Could you check a few things on this model? Use its own coordinates, in mm. A direction names the side the tool comes from. Round coordinates to 2 decimals unless told otherwise and drop trailing zeros. Write each loop counter-clockwise with the first axis right and the second up, starting at its lowest first coordinate (ties: lowest second). Pieces come first, ordered by that corner, then holes. Notation, with made-up numbers: (37.5, -28) - (92.5, -28) arc R30 cw to (92.5, -1) - close; hole circle Ø6 at (34.5, 34). An arc over 180 degrees is marked (long way). Write each question's results on one line, items separated by ' | '. Start each with the question number.
(1) Imagine slicing it at A-A on y = 7. Write out the boundary of the cut face in (x, z).
(2) Imagine slicing it at D-D on y = 15. Write out the boundary of the cut face in (x, z).
(3) Please list where these lines run through material, in increasing order: line 1 (Y direction, x = 11.2, z = 0); line 2 (X direction, y = 21.8, z = 0); line 3 (Z direction, x = 0, y = 22.15). Write a range as [from, to].
(4) On a 3-axis mill with a long thin cutter (end or side, diameter ignored), from which of +Z, -Z, +X, -X, +Y, -Y can I reach the whole of each face in a straight line? I mean faces 1 (the cylindrical face through (10.479, 18.584, -0.314)), 2 (the flat face through (-7, 18, 3)), 3 (the cylindrical face through (11.699, 11.325, 7.815)), 4 (the flat face through (3, 2, -3)), 5 (the flat face through (8, 21, -2.65)). Say none if no direction works.
(5) Thinking about a two-plate mould opening in X: for faces 6 (the flat face through (6, 10, -4)), 7 (the flat face through (5.568, 2.986, -3.155)), 8 (the flat face through (2, 16, 0)), which applies, +X half, -X half, draft (parallel to the pull), parting line (faces both ways), or undercut?
(6) Imagine slicing it at B-B on x = 8. Write out the boundary of the cut face in (y, z).
(7) For P1, Ø0.6, axis at y = 2.5, z = -1.5, coming from the +X side; P2, Ø2.5, axis at y = 19, z = 0.5, coming from the -X side; P3, Ø0.6, axis at x = -6, y = 18.5, coming from the -Z side, each with a flat end and sliding along its axis, tell me the tip position at first contact or that it passes through.
(8) Imagine slicing it at C-C on z = 3. State how many separate pieces and enclosed holes the cut face has, then the cut area to 3 significant figures.
```python
from build123d import *

# Parameters (mm, degrees)
SKETCH1_W                  = 12
SKETCH1_H                  = 13
BOSS_EXTRUDE1_DEPTH        = 19
SKETCH2_R                  = 4
CUT_EXTRUDE1_DEPTH         = 16
CUT_EXTRUDE2_START         = -2
SKETCH3_W                  = 12
SKETCH3_H                  = 13
CUT_EXTRUDE2_DEPTH         = 6
SKETCH5_W                  = 12
SKETCH5_H                  = 13
BOSS_EXTRUDE2_DEPTH        = 5
FILLET1_R                  = 2
FILLET4_R                  = 2
SKETCH21_W                 = 2.5
SKETCH21_H                 = 8
SKETCH21_W_2               = 9
SKETCH21_H_2               = 1.5
BOSS_EXTRUDE4_DEPTH        = 1
FILLET3_R                  = 0.5
FILLET7_R                  = 0.5
FILLET5_R                  = 0.5
SKETCH23_R                 = 4
BOSS_EXTRUDE5_DEPTH        = 1
BOSS_EXTRUDE6_DEPTH        = 13
BOSS_EXTRUDE7_DEPTH        = 25
SKETCH11_W                 = 2.3
SKETCH11_H                 = 5.3
CUT_EXTRUDE4_DEPTH         = 7
SKETCH34_W                 = 13.5
SKETCH34_H                 = 6
CUT_EXTRUDE5_DEPTH         = 15
M2_5_CLEARANCE_HOLE1_D     = 2.9
M2_5_CLEARANCE_HOLE1_DEPTH = 13.378752102
M2_5_CLEARANCE_HOLE1_TIP   = 0.871247898
FILLET8_R                  = 0.4
SKETCH31_R                 = 3.625
SKETCH31_R_2               = 2.625
BOSS_EXTRUDE8_DEPTH        = 2.75
FILLET9_R                  = 1
SKETCH9_R                  = 1
CUT_EXTRUDE6_DEPTH         = 29.889617512
CUT_EXTRUDE8_DEPTH         = 12
FILLET10_R                 = 5
BOSS_EXTRUDE9_DEPTH        = 2


with BuildPart() as part:
    # Sketch1 → Boss-Extrude1 (new body)
    with BuildSketch(Plane(origin=(0, 0, 0), x_dir=(1, 0, 0), z_dir=(0, 1, 0))):
        Rectangle(SKETCH1_W, SKETCH1_H)
    extrude(amount=BOSS_EXTRUDE1_DEPTH)

    # Sketch2 → Cut-Extrude1 (cut)
    with BuildSketch(Plane.XZ):
        with Locations(Location((0, 0, 0), (0, 0, 270))):
            Circle(SKETCH2_R)
    extrude(amount=-CUT_EXTRUDE1_DEPTH, mode=Mode.SUBTRACT)

    # Sketch3 → Cut-Extrude2 (cut)
    with BuildSketch(Plane.XZ.offset(CUT_EXTRUDE2_START)):
        Rectangle(SKETCH3_W, SKETCH3_H)
    extrude(amount=-CUT_EXTRUDE2_DEPTH, mode=Mode.SUBTRACT)


with BuildPart() as cut_extrude2_piece_1:
    # of the separate pieces the step leaves, piece 1, a body of its own (cut_extrude2_pieces)
    add(part.part.solids().sort_by_distance((-6, 8, 6.5))[0])

    # Sketch5 → Boss-Extrude2 (add)
    with BuildSketch(Plane(origin=(0, 19, 0), x_dir=(1, 0, 0), z_dir=(0, 1, 0))):
        Rectangle(SKETCH5_W, SKETCH5_H)
    extrude(amount=BOSS_EXTRUDE2_DEPTH)

    # Fillet1
    fillet1_edges = [cut_extrude2_piece_1.edges().sort_by_distance(p)[0] for p in [
        (-6, 16, -6.5),
        (-6, 16, 6.5),
    ]]
    fillet(fillet1_edges, radius=FILLET1_R)



with BuildPart() as cut_extrude2_piece_2:
    # of the separate pieces the step leaves, piece 2, a body of its own (cut_extrude2_pieces)
    add(part.part.solids().sort_by_distance((-6, 0, 6.5))[0])

    # Fillet4
    fillet4_edges = [cut_extrude2_piece_2.edges().sort_by_distance(p)[0] for p in [
        (-6, 1, 6.5),
        (-6, 1, -6.5),
    ]]
    fillet(fillet4_edges, radius=FILLET4_R)

    # Sketch21 → Boss-Extrude4 (add)
    with BuildSketch(Plane.ZY.offset(6)):
        with Locations((-3.25, 18)):
            Rectangle(SKETCH21_W, SKETCH21_H)
        with Locations((3.25, 18)):
            Rectangle(SKETCH21_W, SKETCH21_H)
        with Locations((0, 0.75)):
            Rectangle(SKETCH21_W_2, SKETCH21_H_2)
    extrude(amount=BOSS_EXTRUDE4_DEPTH)


with BuildPart() as boss_extrude4_piece_1:
    # of the separate pieces the step leaves, piece 1, a body of its own (boss_extrude4_pieces)
    add(cut_extrude2_piece_2.part.solids().sort_by_distance((-4, 0, 6.5))[0])

    # Fillet5
    fillet5_edges = [boss_extrude4_piece_1.edges().sort_by_distance(p)[0] for p in [
        (-7, 0.75, -4.5),
        (-7, 0.75, 4.5),
    ]]
    fillet(fillet5_edges, radius=FILLET5_R)

    # Sketch23 → Boss-Extrude5 (add)
    with BuildSketch(Plane.XZ):
        with BuildLine():
            Line((-7, 4), (-7, -4))
            ThreePointArc((-7, -4), (-6.853553391, -4.353553391), (-6.5, -4.5))
            Line((-6.5, -4.5), (-6, -4.5))
            ThreePointArc((-6, -4.5), (-5.414213562, -5.914213562), (-4, -6.5))
            Line((-4, -6.5), (6, -6.5))
            Line((6, -6.5), (6, 6.5))
            Line((6, 6.5), (-4, 6.5))
            ThreePointArc((-4, 6.5), (-5.414213562, 5.914213562), (-6, 4.5))
            Line((-6, 4.5), (-6.5, 4.5))
            ThreePointArc((-6.5, 4.5), (-6.853553391, 4.353553391), (-7, 4))
        make_face()
        with Locations(Location((0, 0, 0), (0, 0, 270))):
            Circle(SKETCH23_R, mode=Mode.SUBTRACT)
    extrude(amount=BOSS_EXTRUDE5_DEPTH)


with BuildPart() as boss_extrude4_piece_2:
    # of the separate pieces the step leaves, piece 2, a body of its own (boss_extrude4_pieces)
    add(cut_extrude2_piece_2.part.solids().sort_by_distance((-6, 22, -4.5))[0])

    # Fillet7
    fillet7_edges = [boss_extrude4_piece_2.edges().sort_by_distance(p)[0] for p in [
        (-7, 18, -2),
        (-7, 22, -3.25),
        (-7, 18, -4.5),
        (-7, 14, -3.25),
    ]]
    fillet(fillet7_edges, radius=FILLET7_R)


with BuildPart() as boss_extrude4_piece_3:
    # of the separate pieces the step leaves, piece 3, a body of its own (boss_extrude4_pieces)
    add(cut_extrude2_piece_2.part.solids().sort_by_distance((-6, 22, 2))[0])

    # Fillet3
    fillet3_edges = [boss_extrude4_piece_3.edges().sort_by_distance(p)[0] for p in [
        (-7, 22, 3.25),
        (-7, 18, 2),
        (-7, 14, 3.25),
        (-7, 18, 4.5),
    ]]
    fillet(fillet3_edges, radius=FILLET3_R)


with BuildPart() as cut_extrude2_piece_1_1:
    add(cut_extrude2_piece_1.part)

    add(boss_extrude4_piece_1.part)  # Boss-Extrude6 merges Boss-Extrude4 piece 1
    # Sketch26 → Boss-Extrude6 (add, through all)
    with BuildSketch(Plane(origin=(0, 0, -6.5), x_dir=(-1, 0, 0), z_dir=(0, 0, -1))):
        Polygon((-6, 24), (-12, 24), (-12, -1), (-6, -1), (-6, 2), (-9, 2), (-9, 8), (-6, 8), align=None)
    extrude(amount=-BOSS_EXTRUDE6_DEPTH)


    add(boss_extrude4_piece_2.part)  # Boss-Extrude7 merges Boss-Extrude4 piece 2

    add(boss_extrude4_piece_3.part)  # Boss-Extrude7 merges Boss-Extrude4 piece 3
    # Sketch30 → Boss-Extrude7 (add, through all)
    with BuildSketch(Plane(origin=(0, 24, 0), x_dir=(1, 0, 0), z_dir=(0, 1, 0))):
        with BuildLine():
            ThreePointArc((-6, 4.5), (-5.414213562, 5.914213562), (-4, 6.5))
            Line((-4, 6.5), (12, 6.5))
            Line((12, 6.5), (12, 8.1))
            Line((12, 8.1), (-6, 8.1))
            Line((-6, 8.1), (-6, 4.5))
        make_face()
        with BuildLine():
            Line((12, -6.5), (-4, -6.5))
            ThreePointArc((-4, -6.5), (-5.414213562, -5.914213562), (-6, -4.5))
            Line((-6, -4.5), (-6, -8.1))
            Line((-6, -8.1), (12, -8.1))
            Line((12, -8.1), (12, -6.5))
        make_face()
    extrude(amount=-BOSS_EXTRUDE7_DEPTH)

    # Sketch11 → Cut-Extrude4 (cut)
    with BuildSketch(Plane(origin=(0, 24, 0), x_dir=(1, 0, 0), z_dir=(0, 1, 0))):
        with Locations((7.85, 0)):
            Rectangle(SKETCH11_W, SKETCH11_H)
    extrude(amount=-CUT_EXTRUDE4_DEPTH, mode=Mode.SUBTRACT)

    # Sketch34 → Cut-Extrude5 (cut)
    with BuildSketch(Plane.ZY.offset(6)):
        with Locations((0, 5)):
            Rectangle(SKETCH34_W, SKETCH34_H)
    extrude(amount=-CUT_EXTRUDE5_DEPTH, mode=Mode.SUBTRACT)

    # M2.5 Clearance Hole1
    with Locations(Plane(origin=(12, 0, 0), x_dir=(0, 0, -1), z_dir=(1, 0, 0))):
        with Locations((0, 20)):
            Hole(M2_5_CLEARANCE_HOLE1_D / 2, depth=M2_5_CLEARANCE_HOLE1_DEPTH)
            with Locations((0, 0, -(M2_5_CLEARANCE_HOLE1_DEPTH + M2_5_CLEARANCE_HOLE1_TIP / 2))):  # 118° drill point
                Cone(0, M2_5_CLEARANCE_HOLE1_D / 2, M2_5_CLEARANCE_HOLE1_TIP, mode=Mode.SUBTRACT)

    # Fillet8
    fillet8_edges = [cut_extrude2_piece_1_1.edges().sort_by_distance(p)[0] for p in [
        (-6, 11.5, 8.1),
        (-6, 5, 6.75),
        (-6, 5, -6.75),
        (-6, 11.5, -8.1),
    ]]
    fillet(fillet8_edges, radius=FILLET8_R)

    # Sketch31 → Boss-Extrude8 (add)
    with BuildSketch(Plane(origin=(0, 24, 0), x_dir=(1, 0, 0), z_dir=(0, 1, 0))):
        with Locations(Location((0, 0, 0), (0, 0, 90))):
            Circle(SKETCH31_R)
        with Locations(Location((0, 0, 0), (0, 0, 270))):
            Circle(SKETCH31_R_2, mode=Mode.SUBTRACT)
    extrude(amount=BOSS_EXTRUDE8_DEPTH)

    # Fillet9
    fillet9_edges = [cut_extrude2_piece_1_1.edges().sort_by_distance(p)[0] for p in [
        (12, 11.5, 8.1),
        (12, 11.5, -8.1),
    ]]
    fillet(fillet9_edges, radius=FILLET9_R)

    # Sketch9 → Cut-Extrude6 (cut, through all)
    with BuildSketch(Plane(origin=(0, 24, 0), x_dir=(1, 0, 0), z_dir=(0, 1, 0))):
        with Locations(Location((0, 0, 0), (0, 0, 270))):
            Circle(SKETCH9_R)
    extrude(amount=-CUT_EXTRUDE6_DEPTH, mode=Mode.SUBTRACT)

    # Sketch42 → Cut-Extrude8 (cut)
    with BuildSketch(Plane(origin=(12, 0, 0), x_dir=(0, 0, -1), z_dir=(1, 0, 0))):
        with BuildLine():
            Line((-1.5, 16), (1.5, 16))
            ThreePointArc((1.5, 16), (3.267766953, 15.267766953), (4, 13.5))
            Line((4, 13.5), (4, 4.5))
            ThreePointArc((4, 4.5), (3.267766953, 2.732233047), (1.5, 2))
            Line((1.5, 2), (-1.5, 2))
            ThreePointArc((-1.5, 2), (-3.267766953, 2.732233047), (-4, 4.5))
            Line((-4, 4.5), (-4, 13.5))
            ThreePointArc((-4, 13.5), (-3.267766953, 15.267766953), (-1.5, 16))
        make_face()
    extrude(amount=-CUT_EXTRUDE8_DEPTH, mode=Mode.SUBTRACT)

    # Sketch43 → Revolve1 (revolve)
    with BuildSketch(Plane.XY, mode=Mode.PRIVATE) as revolve1_sk:
        Polygon((1, 24), (2.625, 26.75), (2.625, 24), align=None)
    revolve(revolve1_sk.sketch.rotate(Axis((0, 28.9875, 0), (0, -1, 0)), 270), axis=Axis((0, 28.9875, 0), (0, -1, 0)))

    # Fillet10
    fillet10_edges = [cut_extrude2_piece_1_1.edges().sort_by_distance(p)[0] for p in [
        (1, 24, 0),
    ]]
    fillet(fillet10_edges, radius=FILLET10_R)

    # Sketch45 → Boss-Extrude9 (add)
    with BuildSketch(Plane(origin=(0, 2, 0), x_dir=(1, 0, 0), z_dir=(0, 1, 0))):
        Polygon((3.695041723, -6.4), (7.390083446, 0), (3.695041723, 6.4), (9, 6.4), (9, -6.4), align=None)
    extrude(amount=BOSS_EXTRUDE9_DEPTH)


solid = cut_extrude2_piece_1_1.part
```
Response:
1) outline: (-6, -7.7) arc R0.4 ccw to (-5.6, -8.1) - (11, -8.1) arc R1 ccw to (12, -7.1) - (12, -4) - (9, -4) - (9, -6.75) - (-5.6, -6.75) arc R0.4 ccw to (-6, -7.15) - close; (-6, 7.15) arc R0.4 ccw to (-5.6, 6.75) - (9, 6.75) - (9, 4) - (12, 4) - (12, 7.1) arc R1 ccw to (11, 8.1) - (-5.6, 8.1) arc R0.4 ccw to (-6, 7.7) - close
2) outline: (-7, -4) arc R0.5 ccw to (-6.5, -4.5) - (-6, -4.5) - (-6, -7.7) arc R0.4 ccw to (-5.6, -8.1) - (11, -8.1) arc R1 ccw to (12, -7.1) - (12, -3.5) - (1.94, -3.5) arc R4 cw (long way) to (1.94, 3.5) - (12, 3.5) - (12, 7.1) arc R1 ccw to (11, 8.1) - (-5.6, 8.1) arc R0.4 ccw to (-6, 7.7) - (-6, 4.5) - (-6.5, 4.5) arc R0.5 ccw to (-7, 4) - (-7, 2.5) arc R0.5 ccw to (-6.5, 2) - (-6, 2) - (-6, -2) - (-6.5, -2) arc R0.5 ccw to (-7, -2.5) - close
3) line 1: [-1, 2], [16, 18.55], [21.45, 24] | line 2: [-6, -1], [1, 6.7], [9, 12] | line 3: [-8.1, -1], [1, 8.1]
4) face 1: +X | face 2: +Z, -Z, -X, +Y, -Y | face 3: +Z, +X, +Y, -Y | face 4: -X | face 5: +Y
5) face 6: draft | face 7: -X half | face 8: undercut
6) outline: (-1, -8.1) - (24, -8.1) - (24, -2.65) - (17, -2.65) - (17, 2.65) - (24, 2.65) - (24, 8.1) - (-1, 8.1) - close; hole (2, -6.75) - (8, -6.75) - (8, -4) - (13.5, -4) arc R2.5 ccw to (16, -1.5) - (16, 1.5) arc R2.5 ccw to (13.5, 4) - (8, 4) - (8, 6.75) - (2, 6.75) - (2, 6.4) - (4, 6.4) - (4, -6.4) - (2, -6.4) - close
7) P1: x = 9 | P2: x = -6 | P3: z = -8.09
8) separate pieces: 3 | enclosed holes: 0 | area: 243 mm²
